The listing builds one solid part. Answer for the finished solid, in the listing's coordinates (mm). Face numbers are marked on the shaded views. A direction names the side the tool comes from. Round coordinates to 2 decimals unless told otherwise and drop trailing zeros. Write each loop counter-clockwise with the first axis right and the second up, starting at its lowest first coordinate (ties: lowest second). Pieces come first, ordered by that corner, then holes. Notation, with made-up numbers: M -25.5,52 L -15.5,52 A23 ccw -15.5,63 Z; hole C 30,19.5 d10. An arc over 180 degrees is marked long. Write each question's results on one line, items separated by ' | '.
from build123d import *

# Parameters (mm, degrees)
SKETCH1_W                    = 110
SKETCH1_H                    = 50
BASE_FLANGE1_DEPTH           = 6
CUT_EXTRUDE1_DEPTH           = 10
LPATTERN1_COUNT              = 2
LPATTERN1_PITCH              = 57
MIRROR1_COPY_1_DEPTH         = 10
EDGE_FLANGE1_STRIP_W         = 54
EDGE_FLANGE1_STRIP_H         = 6
EDGE_FLANGE1_STRIP_CUT_DEPTH = 50
EDGE_FLANGE1_DEPTH           = 50
EDGE_FLANGE2_STRIP_W         = 54
EDGE_FLANGE2_STRIP_H         = 6
EDGE_FLANGE2_STRIP_CUT_DEPTH = 50
EDGE_FLANGE2_DEPTH           = 50
SKETCH9_R                    = 4.5
CUT_EXTRUDE2_DEPTH           = 10


# Sheet-metal steps are written as plain solids
with BuildPart() as part:
    # Sketch1 → Base-Flange1 (new body)
    with BuildSketch(Plane(origin=(0, 0, 0), x_dir=(0, 0, -1), z_dir=(1, 0, 0))):
        Rectangle(SKETCH1_W, SKETCH1_H)
    extrude(amount=-BASE_FLANGE1_DEPTH)

    # Sketch5 → Cut-Extrude1 (cut)
    with BuildSketch(Plane.ZY.offset(6)):
        with BuildLine():
            Line((-30, 13), (-10, 13))
            ThreePointArc((-10, 13), (-7.5, 10.5), (-10, 8))
            Line((-10, 8), (-30, 8))
            ThreePointArc((-30, 8), (-32.5, 10.5), (-30, 13))
        make_face()
    cut_extrude1 = extrude(amount=-CUT_EXTRUDE1_DEPTH, mode=Mode.SUBTRACT)

    # LPattern1: Cut-Extrude1 ×2
    with Locations(*[(0, 0, i * LPATTERN1_PITCH) for i in range(1, LPATTERN1_COUNT)]):
        add(cut_extrude1, mode=Mode.SUBTRACT)

    # Mirror1: Cut-Extrude1 across plane
    add(cut_extrude1.mirror(Plane.ZX), mode=Mode.SUBTRACT)

    # Mirror1 copy 1 sketch → Mirror1 copy 1 (cut)
    with BuildSketch(Plane(origin=(-6, 0, 57), x_dir=(0, 0, 1), z_dir=(-1, 0, 0))):
        with BuildLine():
            Line((-30, -13), (-10, -13))
            ThreePointArc((-10, -13), (-7.5, -10.5), (-10, -8))
            Line((-10, -8), (-30, -8))
            ThreePointArc((-30, -8), (-32.5, -10.5), (-30, -13))
        make_face()
    extrude(amount=-MIRROR1_COPY_1_DEPTH, mode=Mode.SUBTRACT)

    # Edge-Flange1 strip (across the edge) → Edge-Flange1 strip cut (cut)
    with BuildSketch(Plane(origin=(0, -25, -55), x_dir=(0, 0, 1), z_dir=(0, 1, 0))):
        with Locations((-6, -3)):
            Rectangle(EDGE_FLANGE1_STRIP_W, EDGE_FLANGE1_STRIP_H)
    extrude(amount=EDGE_FLANGE1_STRIP_CUT_DEPTH, mode=Mode.SUBTRACT)

    # Edge-Flange1 section (across the edge) → Edge-Flange1 (add)
    with BuildSketch(Plane(origin=(0, -25, -55), x_dir=(0, 0, 1), z_dir=(0, 1, 0))):
        with BuildLine():
            Line((0, 15), (0, 67))
            Line((0, 67), (6, 67))
            Line((6, 67), (6, 15))
            ThreePointArc((6, 15), (10.393398282, 4.393398282), (21, 0))
            Line((21, 0), (21, -6))
            ThreePointArc((21, -6), (6.150757595, 0.150757595), (0, 15))
        make_face()
    extrude(amount=EDGE_FLANGE1_DEPTH)

    # Edge-Flange2 strip (across the edge) → Edge-Flange2 strip cut (cut)
    with BuildSketch(Plane(origin=(67, 25, -55), x_dir=(-1, 0, 0), z_dir=(0, -1, 0))):
        with Locations((-6, -3)):
            Rectangle(EDGE_FLANGE2_STRIP_W, EDGE_FLANGE2_STRIP_H)
    extrude(amount=EDGE_FLANGE2_STRIP_CUT_DEPTH, mode=Mode.SUBTRACT)

    # Edge-Flange2 section (across the edge) → Edge-Flange2 (add)
    with BuildSketch(Plane(origin=(67, 25, -55), x_dir=(-1, 0, 0), z_dir=(0, -1, 0))):
        with BuildLine():
            Line((0, 15), (0, 104))
            Line((0, 104), (6, 104))
            Line((6, 104), (6, 15))
            ThreePointArc((6, 15), (10.393398282, 4.393398282), (21, 0))
            Line((21, 0), (21, -6))
            ThreePointArc((21, -6), (6.150757595, 0.150757595), (0, 15))
        make_face()
    extrude(amount=EDGE_FLANGE2_DEPTH)

    # Sketch9 → Cut-Extrude2 (cut)
    with BuildSketch(Plane.ZY.offset(-61)):
        with Locations((-94, 0)):
            Circle(SKETCH9_R)
    extrude(amount=-CUT_EXTRUDE2_DEPTH, mode=Mode.SUBTRACT)

    # Mirror2: part across plane


with BuildPart() as part_1:
    add(part.part)
    add(part.part.mirror(Plane(origin=(67, 25, -159), x_dir=(1, 0, 0), z_dir=(0, 0, 1))))


solid = part_1.part
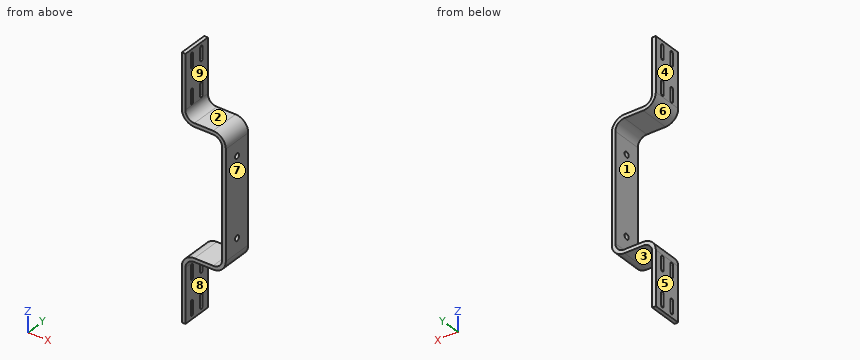
1) Section A-A (x = 33.5) is taken. Determine the outline of the cut face in (y, z), then the cut area to 3 significant figures.
Return value:
outline: M -25,-269 L 25,-269 L 25,-263 L -25,-263 Z; M -25,-55 L 25,-55 L 25,-49 L -25,-49 Z | area: 600 mm²
2) Each of these flat-tipped pins is pushed along its axis until it touches: pin 1 (10 mm diameter, centred on x = 27, y = 14, fed in from +Z); pin 2 (25 mm diameter, centred on x = 23, y = -1.5, fed in from +Z); pin 3 (4 mm diameter, centred on x = 13.5, y = 7.5, fed in from +Z). Where does it stop, or does it pass through?
Return value:
pin 1: z = -49 | pin 2: z = -48.31 | pin 3: z = -48.59
3) Find the intervals of material crossed by line 1 (Y direction, x = 63, z = -224); line 2 (Z direction, x = 24, y = 15.5); line 3 (X direction, y = 22, z = -115.5), in increasing order.
Return value:
line 1: -25 to -4.5, 4.5 to 25 | line 2: -269 to -263, -55 to -49 | line 3: 61 to 67
4) The mould has two halves that part along Z. Classify the marked faces 1, 2, 3 and 4: +Z half, -Z half, draft (parallel to the pull), parting line (faces both ways), or undercut.
Return value:
face 1: undercut | face 2: +Z half | face 3: -Z half | face 4: draft
5) Section B-B (y = 18.5) is taken. Determine the outline of the cut face in (x, z), then the cut area to 3 significant figures.
Return value:
outline: M -6,-373 L 0,-373 L 0,-284 A15 cw 15,-269 L 46,-269 A21 ccw 67,-248 L 67,-70 A21 ccw 46,-49 L 15,-49 A15 cw 0,-34 L 0,55 L -6,55 L -6,-34 A21 ccw 15,-55 L 46,-55 A15 cw 61,-70 L 61,-248 A15 cw 46,-263 L 15,-263 A21 ccw -6,-284 Z | area: 3,190 mm²
6) A tool of negligible diameter and unlimited length cuts with its end or side. For the marked faces 5, 6, 7, 8 and 9, from which of +Z, -Z, +X, -X, +Y, -Y can it reach the whole face along a straight path? Write none if from no direction.
Return value:
face 5: +Z, -Z, -X, +Y, -Y | face 6: -X, +Y, -Y | face 7: +Z, -Z, +X, +Y, -Y | face 8: -Z, +X, +Y, -Y | face 9: +Z, +X, +Y, -Y
